Read the model definition and answer for the solid it produces. Units are mm, in the model's axes. Coordinates: 2 decimals unless noted, no trailing zeros. Write each loop counter-clockwise with the first axis right and the second up, starting at its lowest first coordinate (ties: lowest second). Pieces come first, ordered by that corner, then holes. Notation, with made-up numbers: M 69.5,62.25 L 127.5,62.25 A22 ccw 127.5,101.25 Z; hole C 61.25,-7 d11. An arc over 180 degrees is marked long. Use a Markdown table: item, result. Add a question column.
Autodesk Inventor part; units mm, degrees
ref_plane "YZ Plane" through (0, 0, 0) normal (1, 0, 0) x (0, 1, 0)
ref_plane "XZ Plane" through (0, 0, 0) normal (0, 1, 0) x (-1, 0, 0)
ref_plane "XY Plane" through (0, 0, 0) normal (0, 0, 1) x (1, 0, 0)
sketch "Sketch9" plane through (0, 0, 0) normal (0, 1, 0) x (-1, 0, 0)
  circle A0 centre (0, 0) radius 4
  circle A1 centre (0, 0) radius 5
  dimension "d140" = 8
  dimension "d149" = 10
extrude "Extrusion10" add sketch "Sketch9" along normal blind 26
sketch "Sketch10" plane through (0, 0, 0) normal (0, 0, 1) x (1, 0, 0)
  line L0 (0, 0) -> (0, 6)
  circle A0 centre (0, 6) radius 1
  line L1 (-4, 26) -> (4, 26)
  line L2 (0, 26) -> (0, 20)
  circle A1 centre (0, 20) radius 1
  dimension "d143" = 6
  dimension "d144" = 2
  dimension "d145" = 6
  dimension "d146" = 2
extrude "Extrusion11" cut sketch "Sketch10" along normal mid plane 24
properties part number "airfoil"
Item 1: Determine the mould class of faces 1 (the cylindrical face through (1.08, 12.82, 4.88)), 2 (the cylindrical face through (0.867, 12.818, 3.905)), 3 (the cylindrical face through (-0.8, 5.4, -4.4)) for opening direction Z: pulls with the +Z half, pulls with the -Z half, needs draft (parallel to the pull), parting line crosses it, or undercut.
Item 2: Each of these flat-tipped pins is pushed along its axis until it touches: pin 1 (4 mm diameter, centred on y = 20, z = 3, fed in from +X); pin 2 (1.5 mm diameter, centred on y = 20.5, z = -3.5, fed in from +X); pin 3 (1.8 mm diameter, centred on x = 0, y = 20, fed in from -Z); pin 4 (5 mm diameter, centred on x = 3, y = 5, fed in from +Z). Where does it stop, or does it pass through?
Item 3: Find section A-A on x = -1.75. Give the vertices of the cut face in (y, z), then the cut area to 3 significant figures.
Item 4: Find section B-B on z = -2.75. Give the vertices of the cut face in (x, y).
Item 5: Consider probe 1 along Y at (x, z) = (0, -4.35); probe 2 along Z at (x, y) = (0, 18.75); probe 3 along Z at (x, y) = (-2.25, 5.25). Determine where each line is inside the solid, lowest interval first.
Item 6: Find section D-D on y = 9. Give the vertices of the cut face in (x, z).
Item 7: Find section C-C on x = 0.75. Give the vertices of the cut face in (y, z), then the cut area to 3 significant figures.
Geometry says:
| question | item | result |
|---|---|---|
| 1 | face 1 | parting line crosses it |
| 1 | face 2 | undercut |
| 1 | face 3 | needs draft |
| 2 | pin 1 | stops at x = 4.9 |
| 2 | pin 2 | stops at x = 4.18 |
| 2 | pin 3 | passes through |
| 2 | pin 4 | stops at z = 4.97 |
| 3 | outline | M 0,-4.68 L 26,-4.68 L 26,-3.6 L 0,-3.6 Z; M 0,3.6 L 26,3.6 L 26,4.68 L 0,4.68 Z |
| 3 | area | 56.5 mm2 |
| 4 | outline | M -4.18,0 L -2.9,0 L -2.9,26 L -4.18,26 Z; M 2.9,0 L 4.18,0 L 4.18,26 L 2.9,26 Z |
| 5 | probe 1 | y = 0 to 5, 7 to 19, 21 to 26 |
| 5 | probe 2 | z = -5 to -4, 4 to 5 |
| 5 | probe 3 | z = -4.47 to -3.31, 3.31 to 4.47 |
| 6 | outline | C 0,0 d10; hole C 0,0 d8 |
| 7 | outline | M 0,-4.94 L 5.34,-4.94 L 5.34,-3.93 L 0,-3.93 Z; M 0,3.93 L 5.34,3.93 L 5.34,4.94 L 0,4.94 Z; M 6.66,-4.94 L 19.34,-4.94 L 19.34,-3.93 L 6.66,-3.93 Z; M 6.66,3.93 L 19.34,3.93 L 19.34,4.94 L 6.66,4.94 Z; M 20.66,-4.94 L 26,-4.94 L 26,-3.93 L 20.66,-3.93 Z; M 20.66,3.93 L 26,3.93 L 26,4.94 L 20.66,4.94 Z |
| 7 | area | 47.4 mm2 |
